Input: part model. Units: mm. Frame: model coordinates. A direction names the side the tool comes from. Round coordinates to 2 decimals unless told otherwise and drop trailing zeros. Loops run counter-clockwise (first coordinate to the right, second up) from the corner with the lowest first, then second, coordinate; pieces in that order, holes last. Notation, with made-up numbers: (-18.5, 44.25) - (29.5, 44.25) arc R20 cw to (29.5, 51.25) - close; hole circle Ø7 at (57.5, -25.5). An arc over 180 degrees is marked (long way). One line per question, with ' | ' between items. Start each with the question number.
Item 1: Section D-D, the plane z = 13. Return loops of the section in (x, y) (3 decimals).
Item 2: Section C-C, the plane y = -42.5. Return loops of the section in (x, z).
Item 3: Section A-A, the plane z = 6.5. Return loops of the section in (x, y), plus the area to 3 significant figures.
Item 4: Set-up query: faces 1 (the face through (8, -34.044, 2)), 2 (the face through (8, -37, 4.38)), 3 (the face through (0, -38.594, 15)), 4 (the face through (0, -28, 5)), 5 (the face through (-8, -37, 11.27)). Return all of +Z, -Z, +X, -X, +Y, -Y with unobstructed straight access to the full face (end or side cutting, diameter ignored); none if empty.
Item 5: First-contact query: pin 1 (0.8 mm diameter, centred on x = 7, z = 3, fed in from -Y); pin 2 (4 mm diameter, centred on y = -27, z = 1.5, fed in from -X); pin 3 (2 mm diameter, centred on y = -41, z = 12.5, fed in from -X). Flat tips, straight axial feed; report the tip coordinate or a pass-through.
Item 6: Material intervals for line 1 along Y through (x, z) = (2, 7.25); line 2 along X through (y, z) = (-31.5, 5.25); line 3 along Y through (x, z) = (5.5, 6.25), sorted ascending.
Item 7: Draft query along X for faces 6 (the face through (4.823, -45, 6)), 7 (the face through (-0.052, -37.932, 15.471)), 8 (the face through (-8, -32.329, 6)). Return one class per face: pulls with the +X half, pulls with the -X half, needs draft (parallel to the pull), parting line crosses it, or undercut.
Item 8: Section B-B, the plane x = -4. Return loops of the section in (y, z), plus the area to 3 significant figures.
Autodesk Inventor part; units mm, degrees
ref_plane "Work Plane2" through (0, 0, 0) normal (0, 0, 1) x (1, 0, 0)
ref_plane "Work Plane3" through (0, 0, 0) normal (0, 0, 1) x (1, 0, 0)
ref_plane "Work Plane4" through (0, 0, 0) normal (0, 0, 1) x (1, 0, 0)
sketch "Sketch1" plane through (0, 0, 0) normal (0, 0, 1) x (1, 0, 0)
  line L0 (-6.6921, -30.344) -> (6.8079, -30.344)
  line L1 (6.8079, -30.344) -> (6.8079, -43.844)
  line L2 (6.8079, -43.844) -> (-6.6921, -43.844)
  line L3 (-6.6921, -43.844) -> (-6.6921, -30.344)
  line L4 (-6.6921, -30.344) -> (6.8079, -43.844) construction
  line L5 (6.8079, -30.344) -> (-6.6921, -43.844) construction
  line L6 (-4.7071, -46.444) -> (4.8229, -46.444)
  line L7 (4.8229, -46.444) -> (4.8229, -43.844)
  line L8 (4.8229, -43.844) -> (-4.7071, -43.844)
  line L9 (-4.7071, -43.844) -> (-4.7071, -46.444)
  line L10 (-9.2921, -32.329) -> (-6.6921, -32.329)
  line L11 (-6.6921, -32.329) -> (-6.6921, -41.859)
  line L12 (-6.6921, -41.859) -> (-9.2921, -41.859)
  line L13 (-9.2921, -41.859) -> (-9.2921, -32.329)
  line L14 (6.8079, -34.044) -> (8.3079, -34.044)
  line L15 (8.3079, -34.044) -> (8.3079, -40.144)
  line L16 (8.3079, -40.144) -> (6.8079, -40.144)
  line L17 (6.8079, -40.144) -> (6.8079, -34.044)
  point P0 (0, 0)
  point P1 (0.0579, -37.094)
  point P2 (0.0579, -43.844)
  point P3 (-6.6921, -37.094)
  point P4 (-6.6921, -37.094)
  point P5 (-9.2921, -37.094)
  point P6 (6.8079, -37.094)
  point P7 (8.3079, -37.094)
  point P8 (8.3079, -37.094)
  point P9 (6.8079, -37.094)
  dimension "d0" = 13.5
  dimension "d1" = 13.5
  dimension "d3" = 9.53
  dimension "d4" = 2.6
  dimension "d7" = 2.6
  dimension "d8" = 9.53
  dimension "d19" = 1.5
  dimension "d20" = 6.1
extrude "Extrusion1" add sketch "Sketch1" along normal blind 11.69 contours L0 L1 L2 L3
ref_plane "Work Plane2" through (0, 0, 0) normal (0, 0, 1) x (1, 0, 0)
ref_plane "Work Plane3" through (0, 0, 0) normal (0, 0, 1) x (1, 0, 0)
sketch "Sketch3" plane through (0, 0, 0) normal (0, 0, 1) x (1, 0, 0)
  line L0 (-6.6921, -30.344) -> (6.8079, -30.344)
  line L1 (6.8079, -30.344) -> (6.8079, -43.844)
  line L2 (6.8079, -43.844) -> (-6.6921, -43.844)
  line L3 (-6.6921, -43.844) -> (-6.6921, -30.344)
  line L4 (-6.6921, -30.344) -> (6.8079, -43.844) construction
  line L5 (6.8079, -30.344) -> (-6.6921, -43.844) construction
  line L6 (-4.7071, -46.444) -> (4.8229, -46.444)
  line L7 (4.8229, -46.444) -> (4.8229, -43.844)
  line L8 (4.8229, -43.844) -> (-4.7071, -43.844)
  line L9 (-4.7071, -43.844) -> (-4.7071, -46.444)
  line L10 (-9.2921, -32.329) -> (-6.6921, -32.329)
  line L11 (-6.6921, -32.329) -> (-6.6921, -41.859)
  line L12 (-6.6921, -41.859) -> (-9.2921, -41.859)
  line L13 (-9.2921, -41.859) -> (-9.2921, -32.329)
  line L14 (6.8079, -34.044) -> (8.3079, -34.044)
  line L15 (8.3079, -34.044) -> (8.3079, -40.144)
  line L16 (8.3079, -40.144) -> (6.8079, -40.144)
  line L17 (6.8079, -40.144) -> (6.8079, -34.044)
  point P0 (0, 0)
  point P1 (0, 0)
  point P2 (0.0579, -37.094)
  point P3 (0.0579, -43.844)
  point P4 (-6.6921, -37.094)
  point P5 (-6.6921, -37.094)
  point P6 (-9.2921, -37.094)
  point P7 (6.8079, -37.094)
  point P8 (6.8079, -37.094)
  point P9 (8.3079, -37.094)
  point P10 (8.3079, -37.094)
  dimension "d21" = 13.5
  dimension "d22" = 13.5
  dimension "d23" = 9.53
  dimension "d24" = 2.6
  dimension "d25" = 2.6
  dimension "d26" = 9.53
  dimension "d27" = 1.5
  dimension "d28" = 6.1
extrude "Extrusion2" add sketch "Sketch3" along normal blind 11.27 contours L3 L12 L13 L10 | L2 L7 L6 L9
ref_plane "Work Plane4" through (0, 0, 0) normal (0, 0, 1) x (1, 0, 0)
sketch "Sketch4" plane through (0, 0, 0) normal (0, 0, 1) x (1, 0, 0)
  line L0 (-6.6921, -30.344) -> (6.8079, -30.344)
  line L1 (6.8079, -30.344) -> (6.8079, -43.844)
  line L2 (6.8079, -43.844) -> (-6.6921, -43.844)
  line L3 (-6.6921, -43.844) -> (-6.6921, -30.344)
  line L4 (-6.6921, -30.344) -> (6.8079, -43.844) construction
  line L5 (6.8079, -30.344) -> (-6.6921, -43.844) construction
  line L6 (-4.7071, -46.444) -> (4.8229, -46.444)
  line L7 (4.8229, -46.444) -> (4.8229, -43.844)
  line L8 (4.8229, -43.844) -> (-4.7071, -43.844)
  line L9 (-4.7071, -43.844) -> (-4.7071, -46.444)
  line L10 (-9.2921, -32.329) -> (-6.6921, -32.329)
  line L11 (-6.6921, -32.329) -> (-6.6921, -41.859)
  line L12 (-6.6921, -41.859) -> (-9.2921, -41.859)
  line L13 (-9.2921, -41.859) -> (-9.2921, -32.329)
  line L14 (6.8079, -34.044) -> (8.3079, -34.044)
  line L15 (8.3079, -34.044) -> (8.3079, -40.144)
  line L16 (8.3079, -40.144) -> (6.8079, -40.144)
  line L17 (6.8079, -40.144) -> (6.8079, -34.044)
  point P0 (0, 0)
  point P1 (0, 0)
  point P2 (0, 0)
  point P3 (6.8079, -37.094)
  point P4 (0.0579, -43.844)
  point P5 (-6.6921, -37.094)
  point P6 (0.0579, -37.094)
  point P7 (-6.6921, -37.094)
  point P8 (-9.2921, -37.094)
  point P9 (8.3079, -37.094)
  point P10 (6.8079, -37.094)
  point P11 (8.3079, -37.094)
  dimension "d31" = 13.5
  dimension "d32" = 13.5
  dimension "d33" = 9.53
  dimension "d34" = 2.6
  dimension "d35" = 2.6
  dimension "d36" = 9.53
  dimension "d37" = 1.5
  dimension "d38" = 6.1
extrude "Extrusion3" add sketch "Sketch4" along normal blind 4.38 contours L14 L15 L16 L1
sketch "Sketch5" plane through (0, 0, 11.69) normal (0, 0, 1) x (1, 0, 0)
  line L0 (-6.6921, -30.344) -> (-6.6921, -43.844)
  line L1 (-6.6921, -43.844) -> (6.8079, -43.844)
  line L2 (6.8079, -43.844) -> (6.8079, -30.344)
  line L3 (6.8079, -30.344) -> (-6.6921, -30.344)
  line L4 (6.8079, -30.344) -> (-6.6921, -30.344)
  line L5 (6.8079, -43.844) -> (6.8079, -40.144)
  line L6 (-6.6921, -30.344) -> (-6.6921, -32.329)
  line L7 (1.3808, -38.594) -> (-1.2649, -38.594)
  line L8 (-1.2649, -35.594) -> (1.3808, -35.594)
  arc A0 (1.3808, -38.594) -> (1.3808, -35.594) centre (0.0579, -37.094) ccw
  arc A1 (-1.2649, -35.594) -> (-1.2649, -38.594) centre (0.0579, -37.094) ccw
  circle A2 centre (0.0579, -37.094) radius 0.845
  point P0 (0, 0)
  dimension "d44" = 1.69
extrude "Extrusion4" add sketch "Sketch5" along normal blind 7.67 contours L7 A1 L8 A0
sketch "Sketch6" plane through (0, 0, 0) normal (0, 0, -1) x (-1, 0, 0)
  circle A0 centre (2.4821, -45.984) radius 0.3395
  circle A1 centre (8.832, -39.634) radius 0.3395
  circle A2 centre (8.832, -37.094) radius 0.3395
  circle A3 centre (8.832, -34.554) radius 0.3395
  circle A4 centre (-0.0579, -45.984) radius 0.3395
  circle A5 centre (-2.5979, -45.984) radius 0.3395
  circle A6 centre (-3.2329, -31.4425) radius 0.3395
  circle A7 centre (-3.2329, -26.9975) radius 0.3395
  circle A8 centre (3.117, -31.4425) radius 0.3395
  circle A9 centre (3.1171, -26.9975) radius 0.3395
  point P0 (0, 0)
extrude "Extrusion5" add sketch "Sketch6" along normal blind 1.5
sketch "Sketch7" plane through (0, 0, 0) normal (0, 0, -1) x (-1, 0, 0)
  line L0 (-4.4579, -30.344) -> (4.3421, -30.344)
  line L1 (4.3421, -30.344) -> (4.3421, -25.424)
  line L2 (4.3421, -25.424) -> (-4.4579, -25.424)
  line L3 (-4.4579, -25.424) -> (-4.4579, -30.344)
  line L4 (-6.8079, -30.344) -> (6.6921, -30.344)
  point P0 (0, 0)
  point P1 (-0.0579, -30.344)
  point P2 (-0.0579, -30.344)
  dimension "d49" = 8.8
  dimension "d50" = 4.92
extrude "Extrusion6" add sketch "Sketch7" against normal blind 5
properties part number "Joystick"
Return value:
1) outline: (-1.265, -38.594) - (1.381, -38.594) arc R2 ccw to (1.381, -35.594) - (-1.265, -35.594) arc R2 ccw to start; hole circle Ø1.69 at (0.058, -37.094)
2) outline: (-6.69, 0) - (6.81, 0) - (6.81, 11.69) - (-6.69, 11.69) - close
3) outline: (-9.29, -41.86) - (-6.69, -41.86) - (-6.69, -43.84) - (-4.71, -43.84) - (-4.71, -46.44) - (4.82, -46.44) - (4.82, -43.84) - (6.81, -43.84) - (6.81, -30.34) - (-6.69, -30.34) - (-6.69, -32.33) - (-9.29, -32.33) - close | area: 232 mm2
4) face 1: +Z, -Z, +X, +Y | face 2: +Z, +X, +Y, -Y | face 3: +Z, +X, -X, -Y | face 4: +Z, +X, -X, +Y | face 5: +Z, -X, +Y, -Y
5) pin 1: y = -43.84 | pin 2: x = -4.34 | pin 3: x = -6.69
6) line 1: -46.44 to -30.34 | line 2: -6.69 to 6.81 | line 3: -43.84 to -30.34
7) face 6: pulls with the +X half | face 7: undercut | face 8: needs draft
8) outline: (-46.44, 0) - (-25.42, 0) - (-25.42, 5) - (-30.34, 5) - (-30.34, 11.69) - (-43.84, 11.69) - (-43.84, 11.27) - (-46.44, 11.27) - close | area: 212 mm2
